Geometry check sheet. Reference: the model listing, model coordinates, mm. Round coordinates to 2 decimals unless told otherwise and drop trailing zeros. Order: outer loops, then holes, each group sorted by start corner. A loop starts at its lowest first (then second) coordinate and runs counter-clockwise, first axis right, second up. Notation, with made-up numbers: (38.5, -1) - (74.5, -1) arc R11 ccw to (74.5, 15) - close; hole circle Ø9 at (-40, -22.75). An arc over 180 degrees is marked (long way). One line per question, with ' | ' between items. Start each with the question number.
Q1. Mould release check, pull along Z, two halves, no side actions. Record for faces 1 (the face through (6.35, 1, 3)), 2 (the face through (3.219, 10.403, -165.598)), 3 (the face through (3, -1, -196.85)): +Z half, -Z half, draft (parallel to the pull), parting line (faces both ways), or undercut.
Q2. Sectioned sample at A-A, the plane y = -44.45. Enter the section's corners in (x, z), then the cut area to 3 significant figures.
Q3. Gauge pin test, flat ends, axial feed: P1, Ø6.5, axis at y = -19.05, z = 92.075, coming from the -X side; P2, Ø3, axis at y = 19.05, z = -190.754, coming from the +X side. Record the tip position at first contact, or that the pin passes through.
Q4. Sectioned sample at D-D, the plane z = 5. Enter the section's corners in (x, y).
Q5. Sectioned sample at B-B, the plane z = -152.4. Enter the section's corners in (x, y), then the cut area to 3 significant figures.
Q6. Material ranges on line 1 along Y through (x, z) = (1.75, -152.4); line 2 along Y through (x, z) = (6, -141); line 3 along Y through (x, z) = (5.25, 0), recorded low to high.
Q7. Sectioned sample at C-C, the plane x = 1. Give the number of separate pieces and of enclosed holes in the cut face, then the cut area to 3 significant figures.
```python
from build123d import *

# Parameters (mm, degrees)
SKETCH1_W                                       = 393.7
SKETCH1_H                                       = 127
BOSS_EXTRUDE1_DEPTH                             = 6.35
SKETCH2_R                                       = 14.2875
SKETCH2_R_2                                     = 8.750046
CUT_EXTRUDE1_DEPTH                              = 207.935968357
F_10_CLEARANCE_HOLE1_D                          = 4.9784
CSK_FOR_10_FLAT_HEAD_MACHINE_SCREW2_D           = 5.6134
CSK_FOR_10_FLAT_HEAD_MACHINE_SCREW2_CSINK_D     = 9.779
CSK_FOR_10_FLAT_HEAD_MACHINE_SCREW2_CSINK_ANGLE = 82


with BuildPart() as part:
    # Sketch1 → Boss-Extrude1 (new body)
    with BuildSketch(Plane(origin=(0, 0, 0), x_dir=(0, 0, -1), z_dir=(1, 0, 0))):
        Rectangle(SKETCH1_W, SKETCH1_H)
    extrude(amount=BOSS_EXTRUDE1_DEPTH)

    # Sketch2 → Cut-Extrude1 (cut, through all)
    with BuildSketch(Plane(origin=(6.35, 0, 0), x_dir=(0, 0, -1), z_dir=(1, 0, 0))):
        with Locations((0, 15.875)):
            Circle(SKETCH2_R)
        with Locations((-152.4, 15.875)):
            Circle(SKETCH2_R)
        with Locations((152.4, 15.875)):
            Circle(SKETCH2_R)
        with Locations((-152.4, -44.45)):
            Circle(SKETCH2_R)
        with Locations((152.4, -44.45)):
            Circle(SKETCH2_R)
        with Locations((30.717202021, 31.115)):
            Circle(SKETCH2_R_2)
    extrude(amount=-CUT_EXTRUDE1_DEPTH, mode=Mode.SUBTRACT)

    # #10 Clearance Hole1 (through all)
    with Locations(Plane(origin=(6.35, 0, 0), x_dir=(0, 0, -1), z_dir=(1, 0, 0))):
        with Locations((-190.754, 19.05), (-190.754, -19.05), (190.754, 19.05), (190.754, -19.05)):
            Hole(F_10_CLEARANCE_HOLE1_D / 2)

    # CSK for #10 Flat Head Machine Screw2 (through all)
    with Locations(Plane.ZY):
        with Locations((-92.075, 50.8), (-92.075, -19.05), (92.075, -19.05), (92.075, 50.8)):
            CounterSinkHole(CSK_FOR_10_FLAT_HEAD_MACHINE_SCREW2_D / 2, CSK_FOR_10_FLAT_HEAD_MACHINE_SCREW2_CSINK_D / 2, counter_sink_angle=CSK_FOR_10_FLAT_HEAD_MACHINE_SCREW2_CSINK_ANGLE)


solid = part.part
```
Determined:
1) face 1: draft | face 2: undercut | face 3: -Z half
2) outline: (0, -196.85) - (6.35, -196.85) - (6.35, -166.69) - (0, -166.69) - close; (0, -138.11) - (6.35, -138.11) - (6.35, 138.11) - (0, 138.11) - close; (0, 166.69) - (6.35, 166.69) - (6.35, 196.85) - (0, 196.85) - close | area: 2,140 mm2
3) P1: stops at x = 1.89 | P2: passes through
4) outline: (0, -63.5) - (6.35, -63.5) - (6.35, 2.49) - (0, 2.49) - close; (0, 29.26) - (6.35, 29.26) - (6.35, 63.5) - (0, 63.5) - close
5) outline: (0, -63.5) - (6.35, -63.5) - (6.35, -58.74) - (0, -58.74) - close; (0, -30.16) - (6.35, -30.16) - (6.35, 1.59) - (0, 1.59) - close; (0, 30.16) - (6.35, 30.16) - (6.35, 63.5) - (0, 63.5) - close | area: 444 mm2
6) line 1: y = -63.5 to -58.74, -30.16 to 1.59, 30.16 to 63.5 | line 2: y = -63.5 to -53.06, -35.84 to 7.26, 24.49 to 63.5 | line 3: y = -63.5 to 1.59, 30.16 to 63.5
7) separate pieces: 1 | enclosed holes: 14 | area: 46,300 mm2
